Autodesk Inventor part; units mm, degrees
ref_plane "YZ Plane" through (0, 0, 0) normal (1, 0, 0) x (0, 1, 0)
ref_plane "XZ Plane" through (0, 0, 0) normal (0, 1, 0) x (-1, 0, 0)
ref_plane "XY Plane" through (0, 0, 0) normal (0, 0, 1) x (1, 0, 0)
sketch "Sketch1" plane through (0, 0, 0) normal (0, 1, 0) x (-1, 0, 0)
  line L0 (20, -7.5) -> (-20, -7.5)
  line L1 (-20, -7.5) -> (-20, 7.5)
  line L2 (-20, 7.5) -> (20, 7.5)
  line L3 (20, 7.5) -> (20, -7.5)
  point P0 (0, 0)
  dimension "d0" = 40
  dimension "d1" = 15
  dimension "d2" = 7.5
  dimension "d3" = 20
extrude "Extrusion1" add sketch "Sketch1" along normal blind 65
sketch "Sketch2" plane through (0, 0, 0) normal (0, -1, 0) x (1, 0, 0)
  line L0 (0, 0) -> (0, 0.5)
  line L1 (0, 0.5) -> (8, 0.5)
  line L2 (0, 0.5) -> (-8, 0.5)
  circle A0 centre (-8, 0.5) radius 1.925
  circle A1 centre (8, 0.5) radius 1.925
  dimension "d21" = 0.5
  dimension "d22" = 8
  dimension "d23" = 8
  dimension "d24" = 3.85
  dimension "d25" = 3.85
extrude "Extrusion2" cut sketch "Sketch2" against normal blind 13.7
sketch "Sketch3" plane through (-20, 0, 7.5) normal (0, 0, 1) x (1, 0, 0)
  line L0 (20, 0) -> (20, 45.2)
  circle A0 centre (20, 45.2) radius 8.125
  dimension "d12" = 45.2
  dimension "d13" = 16.25
extrude "Extrusion3" cut sketch "Sketch3" against normal blind 20
properties part number "OmniSupportFront"
Geometry: final body of the model. Coordinates: model frame, mm. A direction names the side the tool comes from. Coordinates: 2 decimals unless noted, no trailing zeros. Order: outer loops, then holes, each group sorted by start corner. A loop starts at its lowest first (then second) coordinate and runs counter-clockwise, first axis right, second up. Notation, with made-up numbers: (-19.5, -9) -> (38.5, -9) arc R10 cw to (38.5, 6) -> close; hole circle Ø3 at (-37, -11). An arc over 180 degrees is marked (long way). Answer in a Markdown table with one row per item.
Item 1: Ray query, L1, parallel to Y at x = 0, z = 2.75 (3 decimals); L2, parallel to Z at x = -8, y = 3.25 (3 decimals); L3, parallel to X at y = 42, z = -4. Return the intervals inside material, ascending.
Return value:
| item | result |
|---|---|
| L1 | y = 0 to 37.075, 53.325 to 65 |
| L2 | z = -7.5 to -1.425, 2.425 to 7.5 |
| L3 | x = -20 to -7.47, 7.47 to 20 |
Item 2: Section C-C on x = 0. Output: boundary loops of the cut face in (y, z) (3 decimals), plus the area to 3 significant figures.
Return value:
| item | result |
|---|---|
| outline | (0, -7.5) -> (37.075, -7.5) -> (37.075, 7.5) -> (0, 7.5) -> close; (53.325, -7.5) -> (65, -7.5) -> (65, 7.5) -> (53.325, 7.5) -> close |
| area | 731 mm² |
Item 3: Section D-D on y = 45.2. Output: boundary loops of the cut face in (x, z) (3 decimals), plus the area to 3 significant figures.
Return value:
| item | result |
|---|---|
| outline | (-20, -7.5) -> (-8.125, -7.5) -> (-8.125, 7.5) -> (-20, 7.5) -> close; (8.125, -7.5) -> (20, -7.5) -> (20, 7.5) -> (8.125, 7.5) -> close |
| area | 356 mm² |
Item 4: Contact query for flat-ended pins moving along their axis: P1, Ø3, axis at x = -8, z = 1, coming from the -Y side; P2, Ø2.5, axis at x = -8, z = 0.5, coming from the -Y side. Output: stop coordinate, or through.
Return value:
| item | result |
|---|---|
| P1 | stops at y = 0 |
| P2 | stops at y = 13.7 |
Item 5: Section A-A on z = 0.5. Output: boundary loops of the cut face in (x, y) (3 decimals).
Return value:
| item | result |
|---|---|
| outline | (-20, 0) -> (-9.925, 0) -> (-9.925, 13.7) -> (-6.075, 13.7) -> (-6.075, 0) -> (6.075, 0) -> (6.075, 13.7) -> (9.925, 13.7) -> (9.925, 0) -> (20, 0) -> (20, 65) -> (-20, 65) -> close; hole circle Ø16.25 at (0, 45.2) |
Item 6: Draft query along Z for faces 1 (the cylindrical face through (6.077, 6.754, 0.585)), 2 (the flat face through (-20, 32, 0)), 3 (the flat face through (0, 32, -7.5)), 4 (the cylindrical face through (-9.923, 6.754, 0.585)). Return one class per face: released by +Z, released by -Z, zero draft, split by the parting line, or undercut.
Return value:
| item | result |
|---|---|
| face 1 | undercut |
| face 2 | zero draft |
| face 3 | released by -Z |
| face 4 | undercut |
Item 7: Access query for faces 5 (the flat face through (8, 13.7, 1)), 6 (the flat face through (0, 65, 0)). Directions: +Z, -Z, +X, -X, +Y, -Y. A direction counts if a zero-diameter tool reaches every point of the face in a straight line with its end or side. Return the directions, or none.
Return value:
| item | result |
|---|---|
| face 5 | -Y |
| face 6 | +Z, -Z, +X, -X, +Y |
Item 8: Section B-B on y = 6. Output: boundary loops of the cut face in (x, z) (3 decimals).
Return value:
| item | result |
|---|---|
| outline | (-20, -7.5) -> (20, -7.5) -> (20, 7.5) -> (-20, 7.5) -> close; hole circle Ø3.85 at (-8, 0.5); hole circle Ø3.85 at (8, 0.5) |
